Verification items for the finished model (mm, model axes). Give positions to 0.01 mm unless a question says otherwise; leave off trailing zeros. Loops run counter-clockwise (first coordinate to the right, second up) from the corner with the lowest first, then second, coordinate; pieces in that order, holes last. Notation, with made-up numbers: (68, 40) - (118, 40) arc R27 ccw to (118, 74) - close; hole circle Ø4 at (13, 78). An arc over 180 degrees is marked (long way). Answer in a Markdown table with one row per item.
Autodesk Fusion 360 part; units mm, degrees
sketch "Skizze1" plane through (0, 0, 0) normal (0, 0, 1) x (1, 0, 0)
  line L0 (0, 0) -> (-28, 0)
  line L1 (-28, 0) -> (-28, 13.6)
  line L2 (-28, 13.6) -> (0, 13.6)
  line L3 (0, 13.6) -> (0, 0)
  line L4 (-28, 6.8) -> (0, 6.8) construction
  circle A0 centre (-24.8, 6.8) radius 1
  circle A1 centre (-3.2, 6.8) radius 1
  line L5 (-14, 13.6) -> (-14, 0) construction
  dimension "d1" = 13.6
  dimension "d2" = 28
  dimension "d5" = 2
  dimension "d6" = 2
  dimension "d7" = 21.6
extrude "Extrusion1" add sketch "Skizze1" along normal blind 23 contours L0 L1 L2 L3 | A0 | A1
extrude "Extrusion2" cut sketch "Skizze1" along normal up to surface (8 mm away) from surface at 15 contours A0 | A1
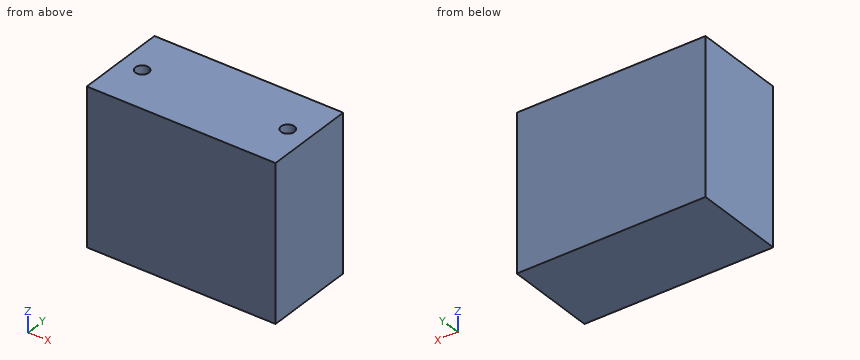
Q1. Go/stop test with a flat-tipped pin: P1, Ø0.6, axis at x = -3, y = 6.5, coming from the +Z side. Record where the tip stops, or that it passes through.
Completed:
| item | result |
|---|---|
| P1 | z = 15 |
Q2. Sectioned sample at A-A (y = 6.8). Record the cut outline in (x, z), and give its area (3 significant figures).
Completed:
| item | result |
|---|---|
| outline | (-28, 0) - (0, 0) - (0, 23) - (-2.2, 23) - (-2.2, 15) - (-4.2, 15) - (-4.2, 23) - (-23.8, 23) - (-23.8, 15) - (-25.8, 15) - (-25.8, 23) - (-28, 23) - close |
| area | 612 mm^2 |
Q3. Thickness scan on line 1 (Y direction, x = -3.2, z = 20.5); line 2 (X direction, y = 6, z = 20.25). Record the ranges inside material, lowest first.
Completed:
| item | result |
|---|---|
| line 1 | 0 to 5.8, 7.8 to 13.6 |
| line 2 | -28 to -25.4, -24.2 to -3.8, -2.6 to 0 |
Q4. Sectioned sample at B-B (x = -3.2). Record the cut outline in (y, z), and give its area (3 significant figures).
Completed:
| item | result |
|---|---|
| outline | (0, 0) - (13.6, 0) - (13.6, 23) - (7.8, 23) - (7.8, 15) - (5.8, 15) - (5.8, 23) - (0, 23) - close |
| area | 297 mm^2 |
